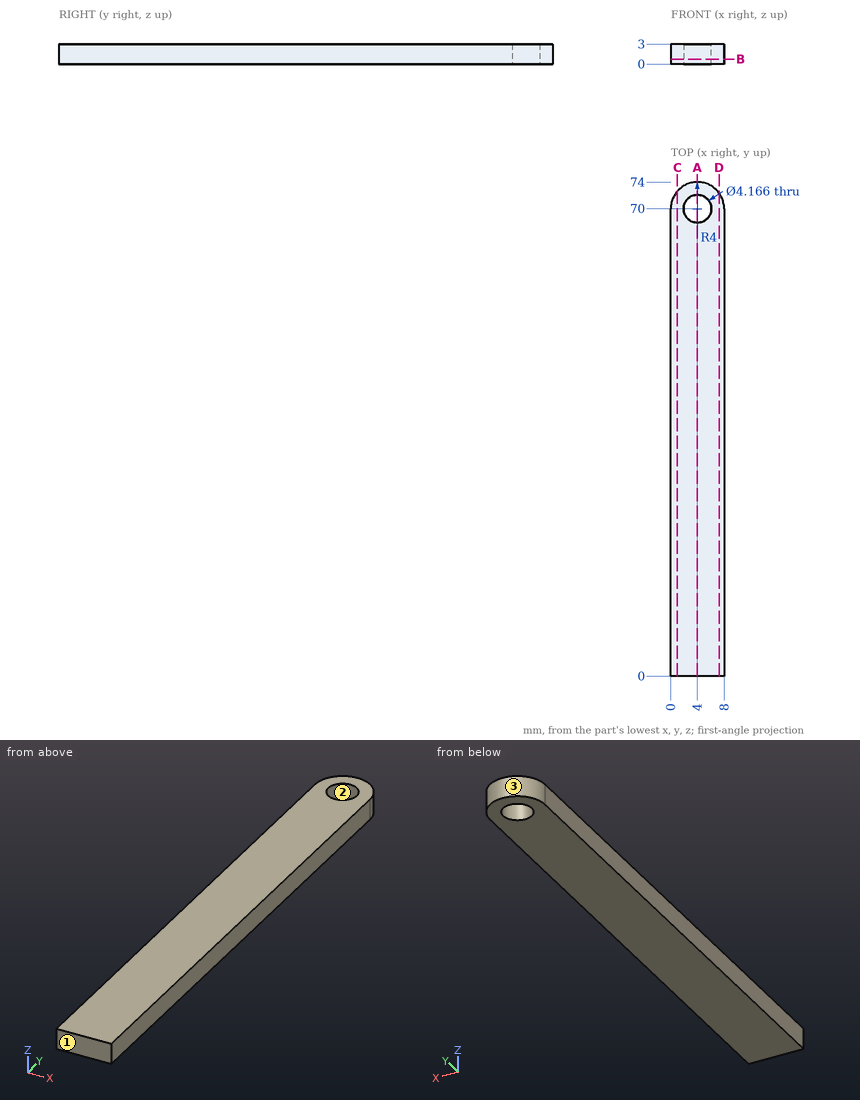
Can you work these out from the drawing? Everything is in mm from the part's minimum corner. Round coordinates to 2 decimals unless told otherwise and drop trailing zeros. Loops run counter-clockwise (first coordinate to the right, second up) from the corner with the lowest first, then second, coordinate; pieces in that order, holes last. Notation, with made-up numbers: (51, 13) - (105, 13) arc R25 ccw to (105, 32) - close; hole circle Ø8 at (-38.75, 50.5). An arc over 180 degrees is marked (long way). Answer in a Markdown table with one row per item. Add a question column.
(1) If we mould it in two halves opening along X, with no side actions, what happens to the marked faces 1, 2 and 3? For each: pulls with the +X half, pulls with the -X half, needs draft (parallel to the pull), parting line crosses it, or undercut.
(2) If we section it at B-B (z = 0.75): Please give me the cut outline in (x, y) (1 decimal).
(3) If we section it at A-A (x = 4): Please give me the cut outline in (y, z).
(4) I need wall thicknesses on line 1 along Y through (x, z) = (4, 2); line 2 along X through (y, z) = (70, 2.2); line 3 along Y through (x, z) = (2.25, 1.5) (1 decimal). Which ranges of each line are inside material? Lowest first, please.
(5) If we section it at C-C (x = 1): Please give me the cut outline in (y, z) (1 decimal), plus the area to 3 significant figures.
(6) If we section it at D-D (x = 7.25): Please give me the cut outline in (y, z), plus the area to 3 significant figures.
Model answer:
| question | item | result |
|---|---|---|
| 1 | face 1 | needs draft |
| 1 | face 2 | undercut |
| 1 | face 3 | parting line crosses it |
| 2 | outline | (0, 0) - (8, 0) - (8, 70) arc R4 ccw to (0, 70) - close; hole circle Ø4.2 at (4, 70) |
| 3 | outline | (0, 0) - (67.92, 0) - (67.92, 3) - (0, 3) - close; (72.08, 0) - (74, 0) - (74, 3) - (72.08, 3) - close |
| 4 | line 1 | y = 0 to 67.92, 72.08 to 74 |
| 4 | line 2 | x = 0 to 1.92, 6.08 to 8 |
| 4 | line 3 | y = 0 to 68.9, 71.1 to 73.6 |
| 5 | outline | (0, 0) - (72.6, 0) - (72.6, 3) - (0, 3) - close |
| 5 | area | 218 mm² |
| 6 | outline | (0, 0) - (72.33, 0) - (72.33, 3) - (0, 3) - close |
| 6 | area | 217 mm² |
